```python
from build123d import *

# Parameters (mm, degrees)
SKETCH1_W           = 17.69
SKETCH1_H           = 20.88
BOSS_EXTRUDE1_DEPTH = 100
SKETCH2_R           = 1.5875
CUT_EXTRUDE1_DEPTH  = 106.78
SKETCH3_R           = 1.5875
CUT_EXTRUDE2_DEPTH  = 100


with BuildPart() as part:
    # Sketch1 → Boss-Extrude1 (new body)
    with BuildSketch(Plane.XY):
        with Locations((8.845, 10.44)):
            Rectangle(SKETCH1_W, SKETCH1_H)
    extrude(amount=BOSS_EXTRUDE1_DEPTH)

    # Sketch2 → Cut-Extrude1 (cut)
    with BuildSketch(Plane(origin=(0, 20.88, 0), x_dir=(1, 0, 0), z_dir=(0, 1, 0))):
        with Locations(Location((8.845, -50, 0), (0, 0, 270))):
            Circle(SKETCH2_R)
    extrude(amount=-CUT_EXTRUDE1_DEPTH, mode=Mode.SUBTRACT)

    # Sketch3 → Cut-Extrude2 (cut)
    with BuildSketch(Plane(origin=(17.69, 0, 0), x_dir=(0, 0, -1), z_dir=(1, 0, 0))):
        with Locations(Location((-87.3, 10.44, 0), (0, 0, 90))):
            Circle(SKETCH3_R)
        with Locations(Location((-12.7, 10.44, 0), (0, 0, 90))):
            Circle(SKETCH3_R)
    extrude(amount=-CUT_EXTRUDE2_DEPTH, mode=Mode.SUBTRACT)


solid = part.part
```
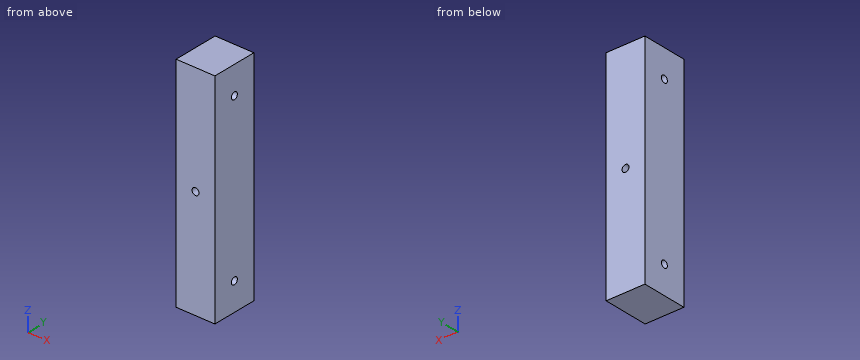
Input: part model. Units: mm. Frame: model coordinates. Give positions to 0.01 mm unless a question says otherwise; leave off trailing zeros. Order: outer loops, then holes, each group sorted by start corner. A loop starts at its lowest first (then second) coordinate and runs counter-clockwise, first axis right, second up.
1. Cut plane C-C (z = 87.3). Return loops of the section in (x, y).
Computed:
outline: (0, 0) - (17.69, 0) - (17.69, 8.85) - (0, 8.85) - close; (0, 12.03) - (17.69, 12.03) - (17.69, 20.88) - (0, 20.88) - close
2. Cut plane A-A (z = 50). Return loops of the section in (x, y).
Computed:
outline: (0, 0) - (7.26, 0) - (7.26, 20.88) - (0, 20.88) - close; (10.43, 0) - (17.69, 0) - (17.69, 20.88) - (10.43, 20.88) - close
3. Pin query (flat end, axial travel): pin 1 Ø1.9 at (y, z) = (10.44, 12.7) entering from -X. Return the tip coordinate at first contact, or that it passes through.
Computed:
pin 1: passes through
4. Cut plane B-B (y = 10). Return loops of the section in (x, z) (1 decimal), and give its area (3 significant figures).
Computed:
outline: (0, 0) - (17.7, 0) - (17.7, 11.2) - (0, 11.2) - close; (0, 14.2) - (17.7, 14.2) - (17.7, 85.8) - (0, 85.8) - close; (0, 88.8) - (17.7, 88.8) - (17.7, 100) - (0, 100) - close; hole circle Ø3.2 at (8.8, 50)
area: 1,650 mm2
5. Line query: probe 1 along Z at (x, y) = (6.75, 10.44); probe 2 along Y at (x, z) = (13.25, 87.3); probe 3 along Z at (x, y) = (15.25, 10). Output: solid intervals per line, ascending.
Computed:
probe 1: z = 0 to 11.11, 14.29 to 85.71, 88.89 to 100
probe 2: y = 0 to 8.85, 12.03 to 20.88
probe 3: z = 0 to 11.17, 14.23 to 85.77, 88.83 to 100
